Part print with two shaded views. Sizes in mm from the minimum x, y, z corner. A direction names the side the tool comes from. Round coordinates to 2 decimals unless told otherwise and drop trailing zeros. Order: outer loops, then holes, each group sorted by start corner. A loop starts at its lowest first (then second) coordinate and runs counter-clockwise, first axis right, second up. Notation, with made-up numbers: M 79,43 L 131,43 A15 ccw 131,54 Z; hole C 48.25,-24 d11. An arc over 180 degrees is marked long. Return JSON: item names as keys, results as strings. Group by question number.
Item 1: Which spindle directions (+Z, -Z, +X, -X, +Y, -Y) get a long thin tool onto all of the face, cutting with end or side? Do the marked faces 1 and 2. Say none if no direction does.
Item 2: Slice it at A-A on y = 22. Give the number of separate pieces and of enclosed holes in the cut face.
Item 3: Slice it at D-D on x = 2.5. Write the cut outline in (y, z).
Item 4: Probe line 1 along X through (y, z) = (9.5, 12.5); line 2 along Z through (x, y) = (32.85, 22); line 3 along X through (y, z) = (6, 2.5). List the from-to ranges inside material, lowest first.
Item 5: Pull direction Y, two halves, no side cores. Call the marked faces 3, 4, 5 and 6: pulls with the +Y half, pulls with the -Y half, needs draft (parallel to the pull), parting line crosses it, or undercut.
Item 6: Pin check, flat tips, straight feed: pin 1 Ø0.6 at (x, z) = (36, 2) entering from -Y; pin 2 Ø1.6 at (x, z) = (36, 1) entering from +Y; pin 3 Ø2.5 at (x, y) = (1.5, 15) entering from +Z; pin 4 Ø3 at (y, z) = (22, 13.75) entering from +X. Stop position of each tip, or through.
Item 7: Slice it at C-C on y = 8. Write the cut outline in (x, z) (1 decimal).
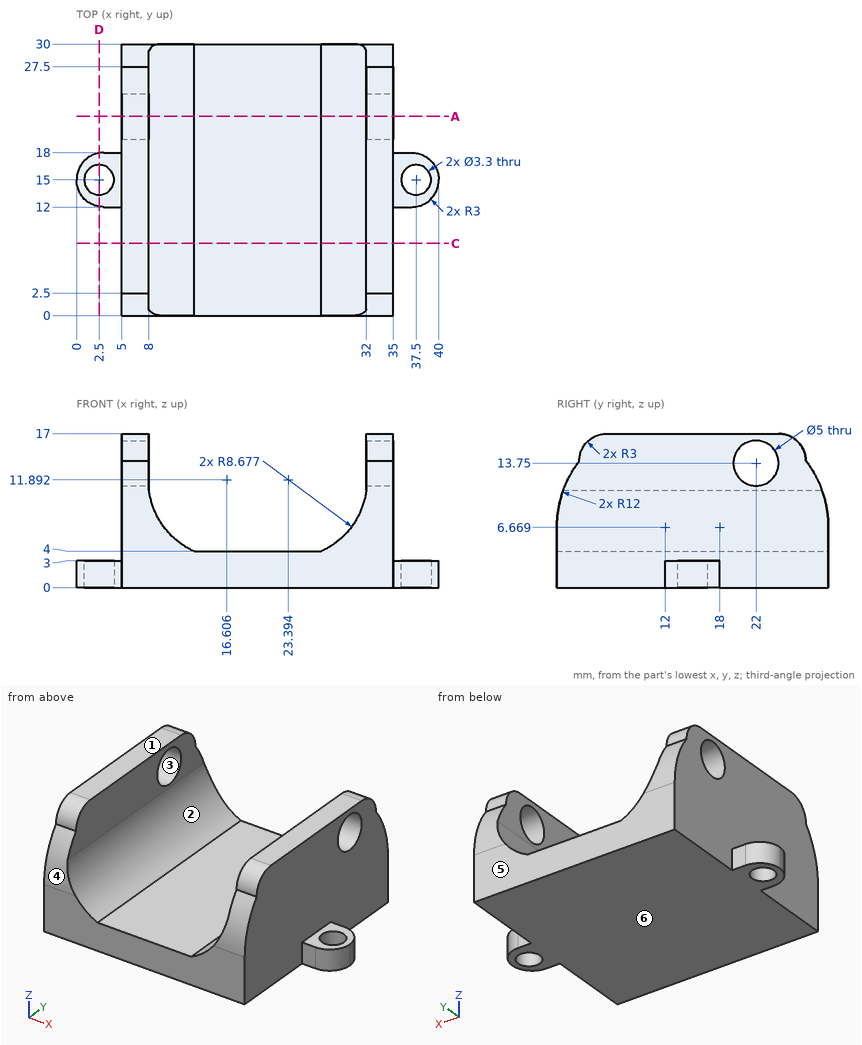
Output values:
{
 "1": {"face 1": "+Z, +X, -X, +Y, -Y", "face 2": "+Z, +Y, -Y"},
 "2": {"separate pieces": "3", "enclosed holes": "0"},
 "3": {"outline": "M 12.04,0 L 13.35,0 L 13.35,3 L 12.04,3 Z; M 16.65,0 L 17.96,0 L 17.96,3 L 16.65,3 Z"},
 "4": {"line 1": "5 to 8, 32 to 35", "line 2": "0 to 11.25, 16.25 to 17", "line 3": "5 to 35"},
 "5": {"face 3": "undercut", "face 4": "pulls with the -Y half", "face 5": "pulls with the +Y half", "face 6": "needs draft"},
 "6": {"pin 1": "y = 12", "pin 2": "y = 18", "pin 3": "z = 3", "pin 4": "through"},
 "7": {"outline": "M 5,0 L 35,0 L 35,17 L 32,17 L 32,10.8 A8.7 cw 27,4 L 13,4 A8.7 cw 8,10.8 L 8,17 L 5,17 Z"}
}
